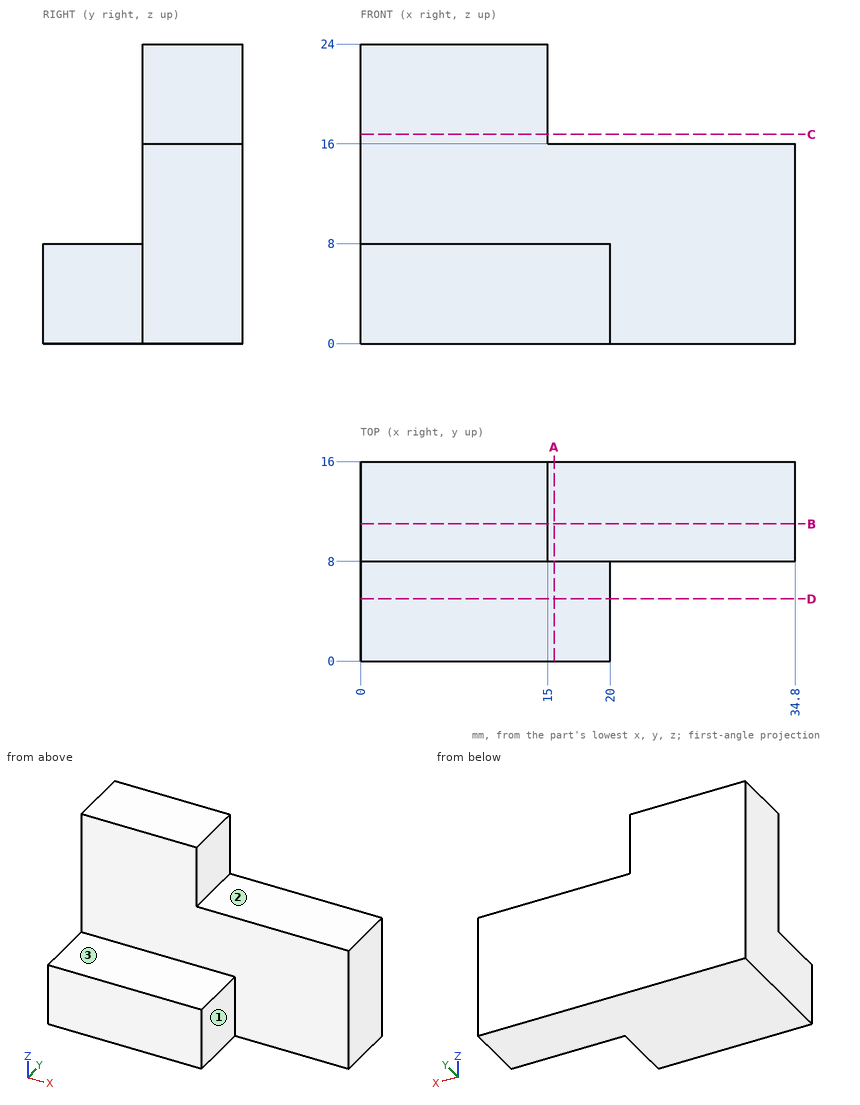
Source: three-view drawing plus pictorial views. Frame: mm from the lowest corner of the part. A direction names the side the tool comes from. Give positions to 0.01 mm unless a question says otherwise; leave off trailing zeros. Write each loop counter-clockwise with the first axis right and the second up, starting at its lowest first coordinate (ties: lowest second). Pieces come first, ordered by that corner, then holes. Notation, with made-up numbers: (22, 7) - (37, 7) arc R20 ccw to (37, 16) - close; hole circle Ø8 at (-31, 89.5). An arc over 180 degrees is marked (long way). Write item = value, one per line. Start each with the question number.
1. First-contact query: pin 1 Ø5 at (x, z) = (5, 17) entering from -Y; pin 2 Ø2.5 at (y, z) = (10.5, 20) entering from +X; pin 3 Ø1 at (x, y) = (29.5, 12.5) entering from +Z. Flat tips, straight axial feed; report the tip coordinate or a pass-through.
2. Section query D-D, the plane y = 5. Output: boundary loops of the cut face in (x, z).
3. Ray query, L1, parallel to Z at x = 29, y = 15; L2, parallel to X at y = 7.5, z = 4.5; L3, parallel to Z at x = 10, y = 6.5. Return the intervals inside material, ascending.
4. Section query C-C, the plane z = 16.75. Output: boundary loops of the cut face in (x, y).
5. Section query A-A, the plane x = 15.5. Output: boundary loops of the cut face in (y, z).
6. Access query for the marked faces 1, 2 and 3. Directions: +Z, -Z, +X, -X, +Y, -Y. A direction counts if a zero-diameter tool reaches every point of the face in a straight line with its end or side. Return the directions, or none.
7. Section query B-B, the plane y = 11. Output: boundary loops of the cut face in (x, z).
Check sheet entries:
q1.pin_1 = 8
q1.pin_2 = 15
q1.pin_3 = 16
q2.outline = (0, 0) - (20, 0) - (20, 8) - (0, 8) - close
q3.L1 = 0 to 16
q3.L2 = 0 to 20
q3.L3 = 0 to 8
q4.outline = (0, 8) - (15, 8) - (15, 16) - (0, 16) - close
q5.outline = (0, 0) - (16, 0) - (16, 16) - (8, 16) - (8, 8) - (0, 8) - close
q6.face_1 = +Z, -Z, +X, -Y
q6.face_2 = +Z, +X, +Y, -Y
q6.face_3 = +Z, +X, -X, -Y
q7.outline = (0, 0) - (34.8, 0) - (34.8, 16) - (15, 16) - (15, 24) - (0, 24) - close
